For this review, use the dimensioned drawing (mm, ordinates from the lowest corner) and the shaded views. A direction names the side the tool comes from. Coordinates: 2 decimals unless noted, no trailing zeros. Loops run counter-clockwise (first coordinate to the right, second up) from the corner with the lowest first, then second, coordinate; pieces in that order, holes last.
1. Take a section at D-D, the plane y = 3. State the section outline as (x, z) points, then the cut area to 3 significant figures.
2. Take a section at C-C, the plane z = 2.65. State the section outline as (x, y) points, then the cut area to 3 significant figures.
3. Clearance check with flat-ended pins moving along their axes: P1, Ø1.5, axis at y = 8.5, z = 3, coming from the +X side; P2, Ø9, axis at x = 8.5, y = 8.5, coming from the -Z side. State where each tip first meets the part, or that it passes through.
4. Mouldability with a two-part tool opening along X and no side actions: class the marked faces 3, 4 and 5 as pulls with the +X half, pulls with the -X half, needs draft (parallel to the pull), parting line crosses it, or undercut.
5. Take a section at A-A, the plane x = 8.5. State the section outline as (y, z) points.
6. To check wall thickness, follow probe 1 along Y at (x, z) = (8.5, 2.15); probe 2 along Z at (x, y) = (1.5, 5.25); probe 3 along X at (y, z) = (12.25, 0.2). State the ranges of each line that lie inside material, in increasing order.
7. Machinability: for the marked faces 1 and 2, which of the approach directions +Z, -Z, +X, -X, +Y, -Y give a long, thin tool a straight path to every point of the face, cutting with its end or side? Answer none if there is none.
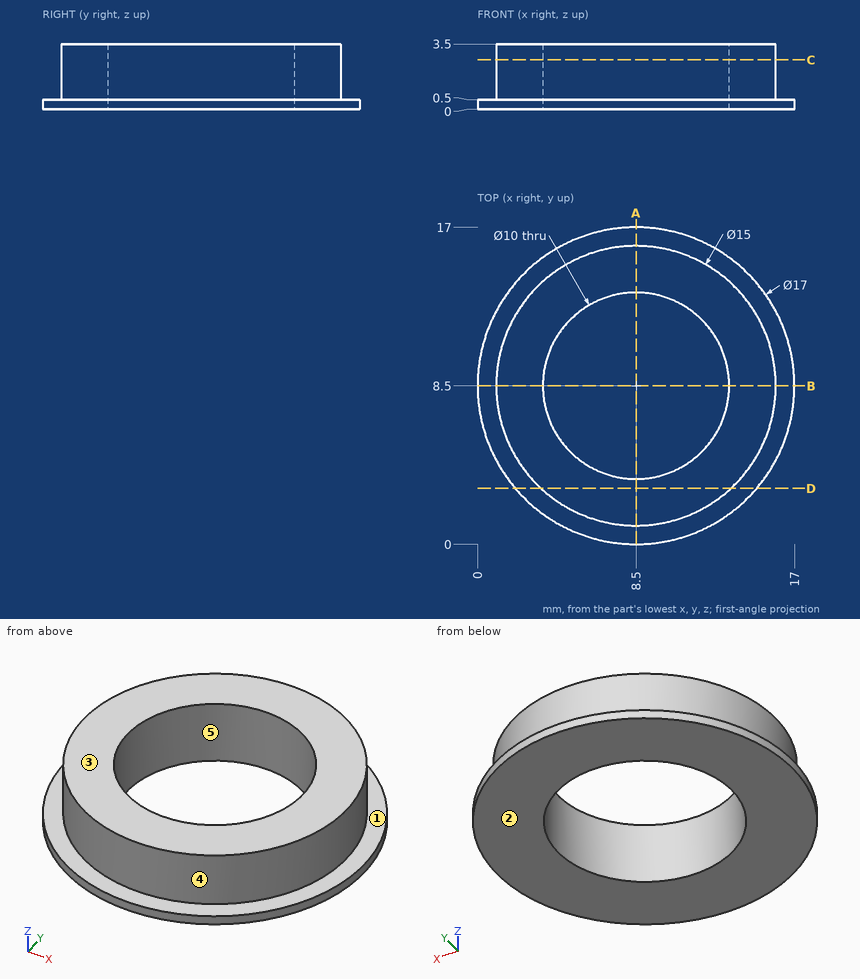
Results list:
1. outline: (2.02, 0) - (14.98, 0) - (14.98, 0.5) - (13.6, 0.5) - (13.6, 3.5) - (3.4, 3.5) - (3.4, 0.5) - (2.02, 0.5) - close
1. area: 37.1 mm2
2. outline: circle Ø15 at (8.5, 8.5); hole circle Ø10 at (8.5, 8.5)
2. area: 98.2 mm2
3. P1: stops at x = 16
3. P2: passes through
4. face 3: needs draft
4. face 4: parting line crosses it
4. face 5: undercut
5. outline: (0, 0) - (3.5, 0) - (3.5, 3.5) - (1, 3.5) - (1, 0.5) - (0, 0.5) - close; (13.5, 0) - (17, 0) - (17, 0.5) - (16, 0.5) - (16, 3.5) - (13.5, 3.5) - close
6. probe 1: y = 1 to 3.5, 13.5 to 16
6. probe 2: z = 0 to 0.5
6. probe 3: x = 0.87 to 5.19, 11.81 to 16.13
7. face 1: +Z
7. face 2: -Z, +X, -X, +Y, -Y
